from build123d import *

# Parameters (mm, degrees)
SKETCH1_W                = 220
SKETCH1_H                = 210
BOSS_EXTRUDE1_DEPTH      = 10
SKETCH2_R                = 65
CUT_EXTRUDE1_DEPTH       = 153.397506541
SKETCH3_R                = 2.25
CUT_EXTRUDE2_DEPTH       = 153.397506541
SKETCH4_R                = 85
CUT_EXTRUDE3_DEPTH       = 3.5
SKETCH5_R                = 4
CUT_EXTRUDE4_DEPTH       = 5
BOSS_EXTRUDE2_DEPTH      = 1.14
BOSS_EXTRUDE2_DEPTH_BACK = 10
SKETCH6_R                = 5.625
CUT_EXTRUDE6_DEPTH       = 153.397506541
CUT_EXTRUDE5_DEPTH       = 146.506305169
SKETCH9_R                = 3.1
CUT_EXTRUDE7_DEPTH       = 11
BOSS_EXTRUDE3_REACH      = 147.423
SKETCH10_W               = 5
SKETCH10_H               = 46.83031672
SKETCH11_R               = 2.5
CUT_EXTRUDE8_DEPTH       = 5
SKETCH12_W               = 64.109170113
SKETCH12_H               = 200.868418625
CUT_EXTRUDE9_DEPTH       = 146.423468683
SKETCH13_R               = 2.5
CUT_EXTRUDE10_DEPTH      = 12
BOSS_EXTRUDE4_DEPTH      = 5
FILLET1_R                = 2.5


with BuildPart() as part:
    # Sketch1 → Boss-Extrude1 (new body)
    with BuildSketch(Plane(origin=(0, 0, 0), x_dir=(1, 0, 0), z_dir=(0, 1, 0))):
        Rectangle(SKETCH1_W, SKETCH1_H)
    extrude(amount=BOSS_EXTRUDE1_DEPTH)

    # Sketch2 → Cut-Extrude1 (cut, through all)
    with BuildSketch(Plane(origin=(0, 10, 0), x_dir=(1, 0, 0), z_dir=(0, 1, 0))):
        with Locations(Location((0, 0, 0), (0, 0, 270))):
            Circle(SKETCH2_R)
    extrude(amount=-CUT_EXTRUDE1_DEPTH, mode=Mode.SUBTRACT)

    # Sketch3 → Cut-Extrude2 (cut, through all)
    with BuildSketch(Plane(origin=(0, 10, 0), x_dir=(1, 0, 0), z_dir=(0, 1, 0))):
        with Locations(Location((70, 60.5, 0), (0, 0, 270))):
            Circle(SKETCH3_R)
        with Locations(Location((-70, 60.5, 0), (0, 0, 270))):
            Circle(SKETCH3_R)
        with Locations(Location((-70, -60.5, 0), (0, 0, 270))):
            Circle(SKETCH3_R)
        with Locations(Location((70, -60.5, 0), (0, 0, 270))):
            Circle(SKETCH3_R)
    extrude(amount=-CUT_EXTRUDE2_DEPTH, mode=Mode.SUBTRACT)

    # Sketch4 → Cut-Extrude3 (cut)
    with BuildSketch(Plane(origin=(0, 10, 0), x_dir=(1, 0, 0), z_dir=(0, 1, 0))):
        with Locations(Location((0, 0, 0), (0, 0, 270))):
            Circle(SKETCH4_R)
    extrude(amount=-CUT_EXTRUDE3_DEPTH, mode=Mode.SUBTRACT)

    # Sketch5 → Cut-Extrude4 (cut)
    with BuildSketch(Plane(origin=(0, 10, 0), x_dir=(1, 0, 0), z_dir=(0, 1, 0))):
        with Locations(Location((70, -60.5, 0), (0, 0, 270))):
            Circle(SKETCH5_R)
        with Locations(Location((-70, -60.5, 0), (0, 0, 270))):
            Circle(SKETCH5_R)
        with Locations(Location((-70, 60.5, 0), (0, 0, 270))):
            Circle(SKETCH5_R)
        with Locations(Location((70, 60.5, 0), (0, 0, 270))):
            Circle(SKETCH5_R)
    extrude(amount=-CUT_EXTRUDE4_DEPTH, mode=Mode.SUBTRACT)

    # Sketch6 → Boss-Extrude2 (add, two sides: drawn at the far end of the back side and taken through both)
    with BuildSketch(Plane(origin=(0, 10, 0), x_dir=(1, 0, 0), z_dir=(0, 1, 0)).offset(-BOSS_EXTRUDE2_DEPTH_BACK)):
        with Locations(Location((-79.674337148, 46, 0), (0, 0, 270))):
            Circle(SKETCH6_R)
        with Locations(Location((-79.674337148, -46, 0), (0, 0, 270))):
            Circle(SKETCH6_R)
    extrude(amount=BOSS_EXTRUDE2_DEPTH + BOSS_EXTRUDE2_DEPTH_BACK)

    # Sketch8 → Cut-Extrude6 (cut, through all)
    with BuildSketch(Plane(origin=(0, 10, 0), x_dir=(1, 0, 0), z_dir=(0, 1, 0))):
        with BuildLine():
            Line((-72.5, -72.5), (-110, -50.849364905))
            Line((-110, -50.849364905), (-110, -105))
            Line((-110, -105), (110, -105))
            Line((110, -105), (110, -50.849364905))
            Line((110, -50.849364905), (72.5, -72.5))
            ThreePointArc((72.5, -72.5), (0, -94.593790725), (-72.5, -72.5))
        make_face()
        with BuildLine():
            Line((-110, 50.849364905), (-72.5, 72.5))
            ThreePointArc((-72.5, 72.5), (0, 94.593790725), (72.5, 72.5))
            Line((72.5, 72.5), (110, 50.849364905))
            Line((110, 50.849364905), (110, 105))
            Line((110, 105), (-110, 105))
            Line((-110, 105), (-110, 50.849364905))
        make_face()
    extrude(amount=-CUT_EXTRUDE6_DEPTH, mode=Mode.SUBTRACT)

    # Sketch7 → Cut-Extrude5 (cut, through all)
    with BuildSketch(Plane(origin=(0, 0, 0), x_dir=(0, 0, -1), z_dir=(1, 0, 0))):
        Polygon((-12.5, 4), (12.5, 4), (12.5, 5.6), (8.1, 10), (-8.1, 10), (-12.5, 5.6), align=None)
    extrude(amount=CUT_EXTRUDE5_DEPTH, mode=Mode.SUBTRACT)

    # Sketch9 → Cut-Extrude7 (cut)
    with BuildSketch(Plane(origin=(0, 11.14, 0), x_dir=(1, 0, 0), z_dir=(0, 1, 0))):
        with Locations(Location((-79.674337148, 46, 0), (0, 0, 270))):
            Circle(SKETCH9_R)
        with Locations(Location((-79.674337148, -46, 0), (0, 0, 270))):
            Circle(SKETCH9_R)
    extrude(amount=-CUT_EXTRUDE7_DEPTH, mode=Mode.SUBTRACT)

    # Sketch10 → Boss-Extrude3 (add, up to next)
    with BuildSketch(Plane(origin=(0, 10, 0), x_dir=(1, 0, 0), z_dir=(0, 1, 0)), mode=Mode.PRIVATE) as boss_extrude3_sk1:
        with Locations((107.5, 0)):
            Rectangle(SKETCH10_W, SKETCH10_H)
    boss_extrude3_tool1 = extrude(boss_extrude3_sk1.sketch, amount=-BOSS_EXTRUDE3_REACH, mode=Mode.PRIVATE) - part.part
    add(boss_extrude3_tool1.solids().sort_by_distance((107.5, 10, 0))[0])

    # Sketch11 → Cut-Extrude8 (cut)
    with BuildSketch(Plane(origin=(110, 0, 0), x_dir=(0, 0, -1), z_dir=(1, 0, 0))):
        with Locations((0, 7)):
            Circle(SKETCH11_R)
    extrude(amount=-CUT_EXTRUDE8_DEPTH, mode=Mode.SUBTRACT)

    # Sketch12 → Cut-Extrude9 (cut, through all)
    with BuildSketch(Plane(origin=(0, 10, 0), x_dir=(1, 0, 0), z_dir=(0, 1, 0))):
        with Locations((-132.054585057, 3.279044808)):
            Rectangle(SKETCH12_W, SKETCH12_H)
    extrude(amount=-CUT_EXTRUDE9_DEPTH, mode=Mode.SUBTRACT)

    # Sketch13 → Cut-Extrude10 (cut)
    with BuildSketch(Plane.ZY.offset(100)):
        with Locations((-40, 5)):
            Circle(SKETCH13_R)
        with Locations((40, 5)):
            Circle(SKETCH13_R)
    extrude(amount=-CUT_EXTRUDE10_DEPTH, mode=Mode.SUBTRACT)

    # Sketch14 → Boss-Extrude4 (add)
    with BuildSketch(Plane(origin=(110, 0, 0), x_dir=(0, 0, -1), z_dir=(1, 0, 0))):
        with BuildLine():
            Line((-5.196152423, 10), (5.196152423, 10))
            ThreePointArc((5.196152423, 10), (0, 13), (-5.196152423, 10))
        make_face()
    extrude(amount=-BOSS_EXTRUDE4_DEPTH)

    # Fillet1
    fillet1_edges = [part.edges().sort_by_distance(p)[0] for p in [
        (107.5, 10, -5.196152423),
        (107.5, 10, 5.196152423),
    ]]
    fillet(fillet1_edges, radius=FILLET1_R)


solid = part.part
The model under review builds one solid part; all positions refer to its coordinate system, in mm. A direction names the side the tool comes from. Round coordinates to 2 decimals unless told otherwise and drop trailing zeros. Loops run counter-clockwise (first coordinate to the right, second up) from the corner with the lowest first, then second, coordinate; pieces in that order, holes last. Notation, with made-up numbers: (40, 26) -> (93, 26) arc R27 cw to (93, 50) -> close; hole circle Ø5 at (39, 9.25). An arc over 180 degrees is marked (long way). Write item = value, one per line. Start each with the question number.
Item 1: To check wall thickness, follow L1, parallel to Y at x = -95.5, z = -40; L2, parallel to X at y = 7.95, z = 60.5; L3, parallel to X at y = 5.5, z = 17. State the ranges of each line that lie inside material, in increasing order.
Item 2: Insertion check: pin 1 (5 mm diameter, centred on x = -70, z = -60.5, fed in from +Y); pin 2 (2.5 mm diameter, centred on y = 4, z = 39.5, fed in from -X); pin 3 (3 mm diameter, centred on x = 53, y = 2.5, fed in from -Z); pin 4 (3.5 mm diameter, centred on x = -70, z = 60.5, fed in from -Y). Each pin has a flat end and moves straight along its axis. Give the tip position at first contact, or say it passes through.
Item 3: Take a section at C-C on z = 46. Give the boundary of the cut face in (x, y).
Item 4: For faces 1 (the cylindrical face through (-94.08, 4.04, -37.69)), 2 (the flat face through (-86.44, 5.07, -64.45)), 3 (the cylindrical face through (-84.665, 10.562, -43.404)), list the 3-axis set-ups (+Z, -Z, +X, -X, +Y, -Y) from which the entire face can be reached by the end or side of a thin tool; tool diameter is ignored.
Item 5: Take a section at B-B on x = 20. Give the boundary of the cut face in (y, z), plus the area to 3 significant figures.
Item 6: Take a section at D-D on x = 61.5. Give the boundary of the cut face in (y, z).
Item 7: Mouldability with a two-part tool opening along Z and no side actions: class faces 4 (the flat face through (-100, 5, 1)), 5 (the flat face through (84, 4, 0)), 6 (the cylindrical face through (-1.08, 5.07, -94.59)) as released by +Z, released by -Z, zero draft, split by the parting line, or undercut.
Item 8: Take a section at A-A on z = 0. Give the boundary of the cut face in (x, y), plus the area to 3 significant figures.
Result:
q1.L1 = 0 to 2.5, 7.5 to 10
q1.L2 = -93.28 to -74, -66 to -59.71, 59.71 to 66, 74 to 93.28
q1.L3 = -100 to -62.74, 62.74 to 110
q2.pin_1 = 5
q2.pin_2 = -88
q2.pin_3 = -83.96
q2.pin_4 = through
q3.outline = (-100, 0) -> (-45.92, 0) -> (-45.92, 6.5) -> (-71.48, 6.5) -> (-71.48, 10) -> (-74.05, 10) -> (-74.05, 11.14) -> (-76.57, 11.14) -> (-76.57, 0.14) -> (-82.77, 0.14) -> (-82.77, 11.14) -> (-85.3, 11.14) -> (-85.3, 10) -> (-100, 10) -> close; (45.92, 0) -> (110, 0) -> (110, 10) -> (71.48, 10) -> (71.48, 6.5) -> (45.92, 6.5) -> close
q4.face_1 = -X
q4.face_2 = -Z, -X, +Y, -Y
q4.face_3 = +Y
q5.outline = (0, -93.05) -> (10, -93.05) -> (10, -82.61) -> (6.5, -82.61) -> (6.5, -61.85) -> (0, -61.85) -> close; (0, 61.85) -> (6.5, 61.85) -> (6.5, 82.61) -> (10, 82.61) -> (10, 93.05) -> (0, 93.05) -> close
q5.area = 479 mm²
q6.outline = (0, -79.13) -> (10, -79.13) -> (10, -58.67) -> (6.5, -58.67) -> (6.5, -21.04) -> (0, -21.04) -> close; (0, 21.04) -> (6.5, 21.04) -> (6.5, 58.67) -> (10, 58.67) -> (10, 79.13) -> (0, 79.13) -> close
q7.face_4 = zero draft
q7.face_5 = undercut
q7.face_6 = released by -Z
q8.outline = (-100, 0) -> (-65, 0) -> (-65, 6.5) -> (-85, 6.5) -> (-85, 10) -> (-100, 10) -> close; (65, 0) -> (110, 0) -> (110, 4.5) -> (105, 4.5) -> (105, 4) -> (65, 4) -> close; (105, 9.5) -> (110, 9.5) -> (110, 13) -> (105, 13) -> close
q8.area = 480 mm²
